Design review of the part shown in the three views and the two pictorial views. Dimensions are in mm from the part's minimum x, y and z. Coordinates: 2 decimals unless noted, no trailing zeros. Order: outer loops, then holes, each group sorted by start corner. A loop starts at its lowest first (then second) coordinate and runs counter-clockwise, first axis right, second up. Notation, with made-up numbers: M 58.5,60.5 L 74.5,60.5 A27 ccw 74.5,77.5 Z; hole C 60,82.5 d2. An arc over 180 degrees is marked long. Use CSV: the item, a comma, the result in double quotes.
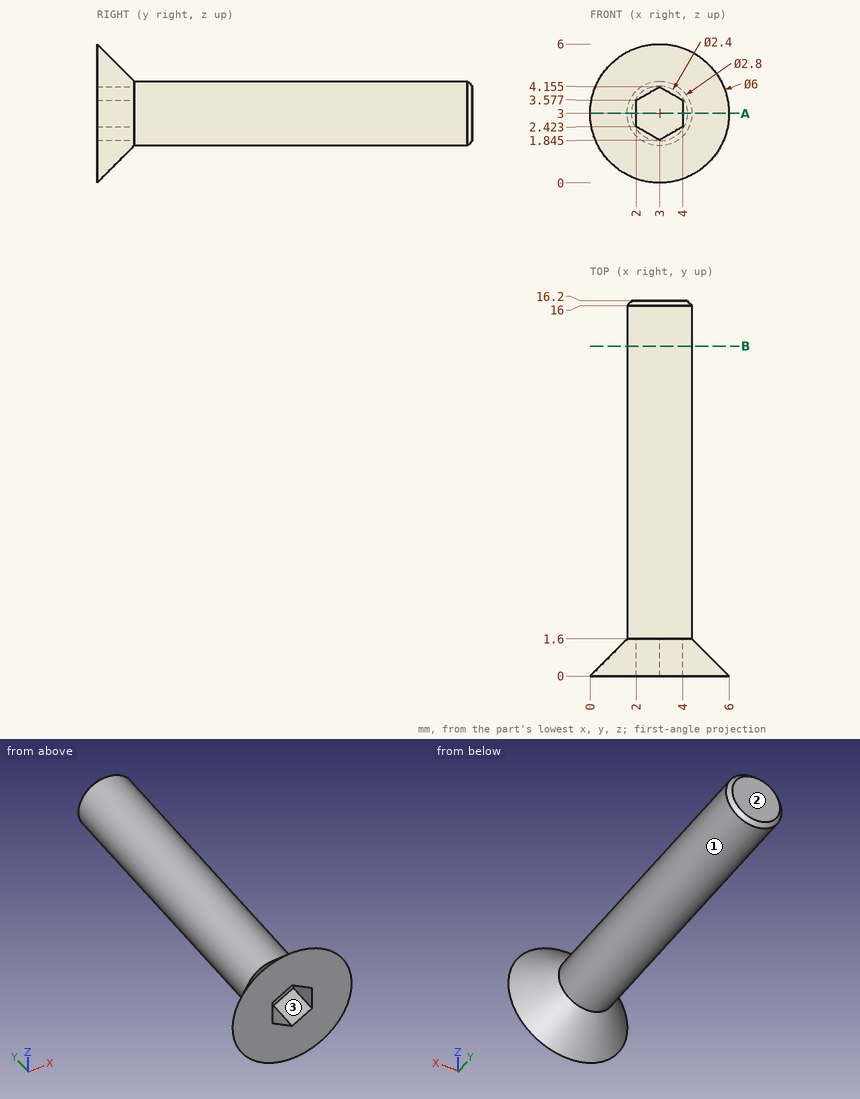
(1) The part is to be moulded in two halves that separate along Z. For the marked faces 1, 2 and 3, say which applies: pulls with the +Z half, pulls with the -Z half, needs draft (parallel to the pull), parting line crosses it, or undercut.
The answers:
face 1,"parting line crosses it"
face 2,"needs draft"
face 3,"undercut"
(2) Wall thickness on probe 1 along Y at (x, z) = (2.8, 2.3); probe 2 along Y at (x, z) = (1.4, 4.15); probe 3 along Z at (x, y) = (4.15, 6.25): over which ranges is each line inside the solid? List them lowest first.
The answers:
probe 1,"y = 1.6 to 16.2"
probe 2,"y = 0 to 1.03"
probe 3,"z = 2.2 to 3.8"
(3) Clearance check with flat-ended pins moving along their axes: P1, Ø1.5, axis at y = 11.5, z = 4, coming from the -X side; P2, Ø2, axis at x = 3.5, y = 4.5, coming from the -Z side; P3, Ø2, axis at x = 1.5, y = 7.5, coming from the +Z side. State where each tip first meets the part, or that it passes through.
The answers:
P1,"stops at x = 1.62"
P2,"stops at z = 1.6"
P3,"stops at z = 4.31"
(4) Add section B-B on y = 14.25. State the section outline as (x, z) points.
The answers:
outline,"C 3,3 d2.8"
(5) Add section A-A on z = 3. State the section outline as (x, y) points.
The answers:
outline,"M 0,0 L 2,0 L 2,1.6 L 4,1.6 L 4,0 L 6,0 L 4.4,1.6 L 4.4,16 L 4.2,16.2 L 1.8,16.2 L 1.6,16 L 1.6,1.6 Z"
